Source: CAD feature listing. Evaluate the final solid. Frame: model axes, mm. Face numbers are marked on the shaded views. A direction names the side the tool comes from. Coordinates: 2 decimals unless noted, no trailing zeros. Order: outer loops, then holes, each group sorted by start corner. A loop starts at its lowest first (then second) coordinate and runs counter-clockwise, first axis right, second up.
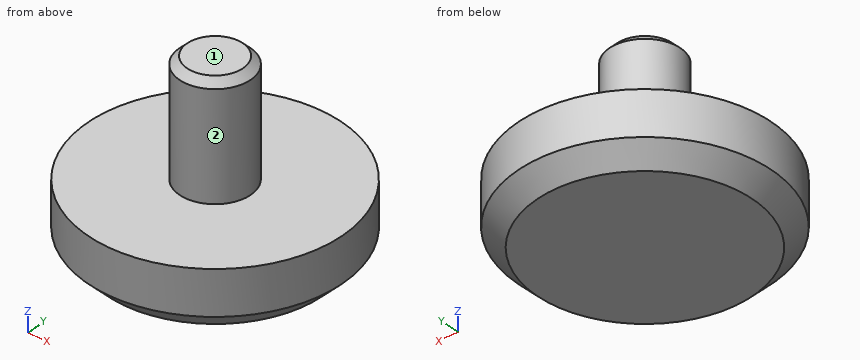
```python
from build123d import *

# Parameters (mm, degrees)
F0_R     = 10
F1_DEPTH = 5
F2_R     = 2.8
F3_DEPTH = 9
F4_SIZE  = 1.5
F5_SIZE  = 0.6


with BuildPart() as f1:
    # F0 (on Top) → F1 (new body)
    with BuildSketch(Plane.XY):
        Circle(F0_R)
    extrude(amount=F1_DEPTH)

    # F2 (on face) → F3 (join)
    with BuildSketch(Plane.XY.offset(5)):
        Circle(F2_R)
    extrude(amount=F3_DEPTH)

    # F4
    f4_edges = [f1.edges().sort_by_distance(p)[0] for p in [
        (-10, 0, 0),
    ]]
    chamfer(f4_edges, length=F4_SIZE)

    # F5
    f5_edges = [f1.edges().sort_by_distance(p)[0] for p in [
        (-2.8, 0, 14),
    ]]
    chamfer(f5_edges, length=F5_SIZE)


solid = f1.part
```
1. Section query C-C on z = 2. Return loops of the section in (x, y), plus the area to 3 significant figures.
Findings:
outline: circle Ø20 at (0, 0)
area: 314 mm2
2. Pin query (flat end, axial travel): P1, Ø5, axis at x = 7.5, y = 6, coming from the +Z side; P2, Ø10, axis at x = 4, y = -2, coming from the +Z side; P3, Ø1, axis at x = 7, z = 2, coming from the -Y side; P4, Ø3, axis at y = -4, z = 3.5, coming from the +X side. Return the tip coordinate at first contact, or that it passes through.
Findings:
P1: stops at z = 5
P2: stops at z = 14
P3: stops at y = -7.6
P4: stops at x = 9.68
3. Section query A-A on y = 0. Return loops of the section in (x, z).
Findings:
outline: (-10, 1.5) - (-8.5, 0) - (8.5, 0) - (10, 1.5) - (10, 5) - (2.8, 5) - (2.8, 13.4) - (2.2, 14) - (-2.2, 14) - (-2.8, 13.4) - (-2.8, 5) - (-10, 5) - close
4. Access query for the marked faces 1 and 2. Directions: +Z, -Z, +X, -X, +Y, -Y. A direction counts if a zero-diameter tool reaches every point of the face in a straight line with its end or side. Return the directions, or none.
Findings:
face 1: +Z, +X, -X, +Y, -Y
face 2: +Z
5. Ray query, line 1 (Z direction, x = -8, y = 1.5); line 2 (X direction, y = 6.5, z = 2); line 3 (Y direction, x = -3, z = 1). Return the intervals inside material, ascending.
Findings:
line 1: z = 0 to 5
line 2: x = -7.6 to 7.6
line 3: y = -9.01 to 9.01
6. Section query D-D on z = 9.25. Return loops of the section in (x, y).
Findings:
outline: circle Ø5.6 at (0, 0)
